Source: CAD feature listing. Evaluate the final solid. Frame: model axes, mm. Round coordinates to 2 decimals unless told otherwise and drop trailing zeros. Write each loop counter-clockwise with the first axis right and the second up, starting at its lowest first coordinate (ties: lowest second). Pieces come first, ordered by that corner, then holes. Notation, with made-up numbers: M -6.75,44 L 12.25,44 A23 cw 12.25,81 Z; hole C 13,63.5 d5. An arc over 180 degrees is marked long. Answer in a Markdown table with one row per item. Add a question column.
Item 1: Contact query for a flat-ended pin moving along its axis: pin 1 (2.5 mm diameter, centred on x = 10, y = 40, fed in from -Z). Output: stop coordinate, or through.
Item 2: Mould query, pull axis Y, two halves, no side actions, for faces 1 (the face through (46.42, 24.26, -1.52)), 2 (the face through (81, 50, -1)), 3 (the face through (0, 25, -1)). Classes: released by +Y, released by -Y, zero draft, split by the parting line, or undercut.
Item 3: Cut plane B-B on y = 45. Return loops of the section in (x, z), and give its area (3 significant figures).
Item 4: Material intervals for probe 1 along X at (y, z) = (45, -2.3); probe 2 along X at (y, z) = (10, -1.75); probe 3 along Y at (x, z) = (115, -1.5), sorted ascending.
Item 5: Cut plane A-A on x = 45. Return loops of the section in (y, z).
Item 6: Cut plane C-C on x = 130. Return loops of the section in (y, z), and give its area (3 significant figures).
Autodesk Inventor part; units mm, degrees
ref_plane "YZ Plane" through (0, 0, 0) normal (1, 0, 0) x (0, 1, 0)
ref_plane "XZ Plane" through (0, 0, 0) normal (0, 1, 0) x (-1, 0, 0)
ref_plane "XY Plane" through (0, 0, 0) normal (0, 0, 1) x (1, 0, 0)
sketch "スケッチ1" plane through (0, 0, 0) normal (0, 0, 1) x (1, 0, 0)
  line L0 (0, 0) -> (160, 0)
  line L1 (160, 0) -> (160, 50)
  line L2 (160, 50) -> (0, 50)
  line L3 (0, 50) -> (0, 0)
  dimension "d0" = 160
  dimension "d1" = 50
extrude "押し出し1" add sketch "スケッチ1" against normal blind 3
sketch "スケッチ2" plane through (0, 0, 0) normal (0, 0, 1) x (1, 0, 0)
  line L0 (160, 50) -> (0, 50)
  line L1 (160, 0) -> (160, 50)
  line L2 (0, 50) -> (0, 0)
  line L3 (0, 0) -> (160, 0)
  point P0 (135, 45)
  point P1 (135, 25)
  point P2 (25, 45)
  point P3 (25, 25)
  point P4 (115, 45)
  point P5 (115, 25)
  point P6 (45, 45)
  point P7 (45, 25)
  point P8 (150, 40)
  point P9 (150, 10)
  point P10 (10, 40)
  point P11 (10, 10)
  dimension "d4" = 5
  dimension "d5" = 25
  dimension "d6" = 20
  dimension "d7" = 5
  dimension "d8" = 25
  dimension "d9" = 20
  dimension "d10" = 20
  dimension "d11" = 20
  dimension "d12" = 10
  dimension "d13" = 10
  dimension "d14" = 10
  dimension "d15" = 10
  dimension "d16" = 20
  dimension "d17" = 5
  dimension "d18" = 5
  dimension "d19" = 20
hole "穴1" at (135, 45, 0) at (135, 25, 0) at (25, 45, 0) at (25, 25, 0) at (115, 45, 0) at (115, 25, 0) at (45, 45, 0) at (45, 25, 0) at (150, 40, 0) at (150, 10, 0) at (10, 40, 0) at (10, 10, 0) direction (0, 0, -1) diameter 3.2 end through all
sketch "スケッチ3" plane through (0, 0, 0) normal (0, 0, 1) x (1, 0, 0)
  line L0 (0, 0) -> (160, 0)
  line L1 (0, 50) -> (0, 0)
  line L2 (160, 0) -> (160, 50)
  point P0 (30, 10)
  point P1 (130, 10)
  dimension "d27" = 10
  dimension "d28" = 30
  dimension "d29" = 10
  dimension "d30" = 30
hole "穴2" at (30, 10, 0) at (130, 10, 0) direction (0, 0, -1) diameter 3.2 end through all
properties part number "frontPlate" material "アルミニウム 6061"
Results below:
| question | item | result |
|---|---|---|
| 1 | pin 1 | through |
| 2 | face 1 | undercut |
| 2 | face 2 | released by +Y |
| 2 | face 3 | zero draft |
| 3 | outline | M 0,-3 L 23.4,-3 L 23.4,0 L 0,0 Z; M 26.6,-3 L 43.4,-3 L 43.4,0 L 26.6,0 Z; M 46.6,-3 L 113.4,-3 L 113.4,0 L 46.6,0 Z; M 116.6,-3 L 133.4,-3 L 133.4,0 L 116.6,0 Z; M 136.6,-3 L 160,-3 L 160,0 L 136.6,0 Z |
| 3 | area | 442 mm2 |
| 4 | probe 1 | 0 to 23.4, 26.6 to 43.4, 46.6 to 113.4, 116.6 to 133.4, 136.6 to 160 |
| 4 | probe 2 | 0 to 8.4, 11.6 to 28.4, 31.6 to 128.4, 131.6 to 148.4, 151.6 to 160 |
| 4 | probe 3 | 0 to 23.4, 26.6 to 43.4, 46.6 to 50 |
| 5 | outline | M 0,-3 L 23.4,-3 L 23.4,0 L 0,0 Z; M 26.6,-3 L 43.4,-3 L 43.4,0 L 26.6,0 Z; M 46.6,-3 L 50,-3 L 50,0 L 46.6,0 Z |
| 6 | outline | M 0,-3 L 8.4,-3 L 8.4,0 L 0,0 Z; M 11.6,-3 L 50,-3 L 50,0 L 11.6,0 Z |
| 6 | area | 140 mm2 |
